The listing builds one solid part. Answer for the finished solid, in the listing's coordinates (mm). A direction names the side the tool comes from. Round coordinates to 2 decimals unless told otherwise and drop trailing zeros. Loops run counter-clockwise (first coordinate to the right, second up) from the corner with the lowest first, then second, coordinate; pieces in that order, holes last. Notation, with made-up numbers: (-32.5, 75) -> (-2.5, 75) arc R20 cw to (-2.5, 107) -> close; hole circle Ø1 at (3.5, 62). An arc over 180 degrees is marked (long way). Use a Markdown table: item, result. Add a question column.
Q1. Given pin 1 Ø7 at (x, z) = (1.5, -4.5) entering from -Y; pin 2 Ø6.5 at (x, z) = (1.5, 168.5) entering from +Y; pin 3 Ø5 at (x, z) = (0.5, 169) entering from -Y, each flat-ended and moving along its own axis, determine where each tip first touches the part or whether it passes through.
Q2. Section B-B on z = 98.5 is taken. Give the vertices of the cut face in (x, y).
Q3. Section A-A on z = -5 is taken. Give the vertices of the cut face in (x, y), then the cut area to 3 significant figures.
Q4. Consider line 1 (Z direction, x = -3.5, y = -7); line 2 (X direction, y = 1.35, z = 167.5); line 3 (Y direction, x = 0.25, z = 140.5). Determine where each line is inside the solid, lowest interval first.
Q5. Which of the six approach directions +Z, -Z, +X, -X, +Y, -Y give full straight-line access (tool end or side, diameter ignored) to faces 5 (the flat face through (0, 4.973, -2)), 6 (the flat face through (0, -4.852, 112)), 7 (the flat face through (7.768, 1, 158))?
Q6. For a pull along Z with two mould halves and no side action, classify faces 1 (the flat face through (0, 1, -9)), 2 (the flat face through (-3, 5, 161)), 3 (the flat face through (0, 8, 70)), 4 (the flat face through (0, 8.648, 158)) as released by +Z, released by -Z, zero draft, split by the parting line, or undercut.
from build123d import *

# Parameters (mm, degrees)
SKETCH2_W           = 23
SKETCH2_H           = 19
BOSS_EXTRUDE1_DEPTH = 70
SKETCH3_W           = 10
SKETCH3_H           = 8
BOSS_EXTRUDE2_DEPTH = 9
SKETCH4_R           = 2
CUT_EXTRUDE1_DEPTH  = 73.156975517
SKETCH5_W           = 12
SKETCH5_H           = 12
BOSS_EXTRUDE3_DEPTH = 85
SKETCH6_W           = 15
SKETCH6_H           = 15
BOSS_EXTRUDE4_DEPTH = 6
BOSS_EXTRUDE5_DEPTH = 10
CUT_EXTRUDE2_START  = -6
CUT_EXTRUDE2_DEPTH  = 6
SKETCH9_R           = 2
CUT_EXTRUDE3_DEPTH  = 172.816281943


with BuildPart() as part:
    # Sketch2 → Boss-Extrude1 (new body)
    with BuildSketch(Plane.XY):
        with Locations((-0.231543624, 1.473154362)):
            Rectangle(SKETCH2_W, SKETCH2_H)
    extrude(amount=BOSS_EXTRUDE1_DEPTH)

    # Sketch3 → Boss-Extrude2 (add)
    with BuildSketch(Plane(origin=(0, 0, 0), x_dir=(-1, 0, 0), z_dir=(0, 0, -1))):
        with Locations((-0.268456376, 0.973154362)):
            Rectangle(SKETCH3_W, SKETCH3_H)
    extrude(amount=BOSS_EXTRUDE2_DEPTH)

    # Sketch4 → Cut-Extrude1 (cut, through all)
    with BuildSketch(Plane(origin=(0, 4.973154362, 0), x_dir=(1, 0, 0), z_dir=(0, 1, 0))):
        with Locations(Location((0.268456376, 5, 0), (0, 0, 180))):
            Circle(SKETCH4_R)
    extrude(amount=-CUT_EXTRUDE1_DEPTH, mode=Mode.SUBTRACT)

    # Sketch5 → Boss-Extrude3 (add)
    with BuildSketch(Plane.XY.offset(70)):
        with Locations((0.268456376, 1.148154362)):
            Rectangle(SKETCH5_W, SKETCH5_H)
    extrude(amount=BOSS_EXTRUDE3_DEPTH)

    # Sketch6 → Boss-Extrude4 (add)
    with BuildSketch(Plane.XY.offset(155)):
        with Locations((0.268456376, 1.148154362)):
            Rectangle(SKETCH6_W, SKETCH6_H)
    extrude(amount=BOSS_EXTRUDE4_DEPTH)

    # Sketch7 → Boss-Extrude5 (add)
    with BuildSketch(Plane.XY.offset(161)):
        with BuildLine():
            ThreePointArc((-4.231543624, 1.148154362), (-2.91352414, -2.033826153), (0.268456376, -3.351845638))
            Line((0.268456376, -3.351845638), (0.268456376, 1.148154362))
            Line((0.268456376, 1.148154362), (-4.231543624, 1.148154362))
        make_face()
        with BuildLine():
            Line((0.268456376, 1.148154362), (0.268456376, -3.351845638))
            ThreePointArc((0.268456376, -3.351845638), (3.450436891, -2.033826153), (4.768456376, 1.148154362))
            Line((4.768456376, 1.148154362), (0.268456376, 1.148154362))
        make_face()
        with BuildLine():
            Line((-4.231543624, 1.148154362), (0.268456376, 1.148154362))
            Line((0.268456376, 1.148154362), (0.268456376, 5.648154362))
            ThreePointArc((0.268456376, 5.648154362), (-2.91352414, 4.330134878), (-4.231543624, 1.148154362))
        make_face()
        with BuildLine():
            Line((0.268456376, 5.648154362), (0.268456376, 1.148154362))
            Line((0.268456376, 1.148154362), (4.768456376, 1.148154362))
            ThreePointArc((4.768456376, 1.148154362), (3.450436891, 4.330134878), (0.268456376, 5.648154362))
        make_face()
        with BuildLine():
            ThreePointArc((-4.231543624, 1.148154362), (-2.91352414, -2.033826153), (0.268456376, -3.351845638))
            Line((0.268456376, -3.351845638), (0.268456376, 1.148154362))
            Line((0.268456376, 1.148154362), (-4.231543624, 1.148154362))
        make_face()
        with BuildLine():
            Line((0.268456376, 1.148154362), (0.268456376, -3.351845638))
            ThreePointArc((0.268456376, -3.351845638), (3.450436891, -2.033826153), (4.768456376, 1.148154362))
            Line((4.768456376, 1.148154362), (0.268456376, 1.148154362))
        make_face()
        with BuildLine():
            Line((-4.231543624, 1.148154362), (0.268456376, 1.148154362))
            Line((0.268456376, 1.148154362), (0.268456376, 5.648154362))
            ThreePointArc((0.268456376, 5.648154362), (-2.91352414, 4.330134878), (-4.231543624, 1.148154362))
        make_face()
        with BuildLine():
            Line((0.268456376, 5.648154362), (0.268456376, 1.148154362))
            Line((0.268456376, 1.148154362), (4.768456376, 1.148154362))
            ThreePointArc((4.768456376, 1.148154362), (3.450436891, 4.330134878), (0.268456376, 5.648154362))
        make_face()
        with BuildLine():
            ThreePointArc((-4.231543624, 1.148154362), (-2.91352414, -2.033826153), (0.268456376, -3.351845638))
            Line((0.268456376, -3.351845638), (0.268456376, 1.148154362))
            Line((0.268456376, 1.148154362), (-4.231543624, 1.148154362))
        make_face()
        with BuildLine():
            Line((0.268456376, 1.148154362), (0.268456376, -3.351845638))
            ThreePointArc((0.268456376, -3.351845638), (3.450436891, -2.033826153), (4.768456376, 1.148154362))
            Line((4.768456376, 1.148154362), (0.268456376, 1.148154362))
        make_face()
        with BuildLine():
            Line((-4.231543624, 1.148154362), (0.268456376, 1.148154362))
            Line((0.268456376, 1.148154362), (0.268456376, 5.648154362))
            ThreePointArc((0.268456376, 5.648154362), (-2.91352414, 4.330134878), (-4.231543624, 1.148154362))
        make_face()
        with BuildLine():
            Line((0.268456376, 5.648154362), (0.268456376, 1.148154362))
            Line((0.268456376, 1.148154362), (4.768456376, 1.148154362))
            ThreePointArc((4.768456376, 1.148154362), (3.450436891, 4.330134878), (0.268456376, 5.648154362))
        make_face()
        with BuildLine():
            ThreePointArc((-4.231543624, 1.148154362), (-2.91352414, -2.033826153), (0.268456376, -3.351845638))
            Line((0.268456376, -3.351845638), (0.268456376, 1.148154362))
            Line((0.268456376, 1.148154362), (-4.231543624, 1.148154362))
        make_face()
        with BuildLine():
            Line((0.268456376, 1.148154362), (0.268456376, -3.351845638))
            ThreePointArc((0.268456376, -3.351845638), (3.450436891, -2.033826153), (4.768456376, 1.148154362))
            Line((4.768456376, 1.148154362), (0.268456376, 1.148154362))
        make_face()
        with BuildLine():
            Line((-4.231543624, 1.148154362), (0.268456376, 1.148154362))
            Line((0.268456376, 1.148154362), (0.268456376, 5.648154362))
            ThreePointArc((0.268456376, 5.648154362), (-2.91352414, 4.330134878), (-4.231543624, 1.148154362))
        make_face()
        with BuildLine():
            Line((0.268456376, 5.648154362), (0.268456376, 1.148154362))
            Line((0.268456376, 1.148154362), (4.768456376, 1.148154362))
            ThreePointArc((4.768456376, 1.148154362), (3.450436891, 4.330134878), (0.268456376, 5.648154362))
        make_face()
    extrude(amount=BOSS_EXTRUDE5_DEPTH)

    # Sketch8 → Cut-Extrude2 (cut)
    with BuildSketch(Plane.XY.offset(171).offset(CUT_EXTRUDE2_START)):
        with BuildLine():
            Line((-3.293495336, 3.898154362), (0.268456376, 3.898154362))
            Line((0.268456376, 3.898154362), (0.268456376, 5.648154362))
            ThreePointArc((0.268456376, 5.648154362), (-1.715857107, 5.187027968), (-3.293495336, 3.898154362))
        make_face()
        with BuildLine():
            Line((0.268456376, 5.648154362), (0.268456376, 3.898154362))
            Line((0.268456376, 3.898154362), (3.830408088, 3.898154362))
            ThreePointArc((3.830408088, 3.898154362), (2.252769859, 5.187027968), (0.268456376, 5.648154362))
        make_face()
        with BuildLine():
            Line((-3.293495336, 3.898154362), (0.268456376, 3.898154362))
            Line((0.268456376, 3.898154362), (0.268456376, 5.648154362))
            ThreePointArc((0.268456376, 5.648154362), (-1.715857107, 5.187027968), (-3.293495336, 3.898154362))
        make_face()
        with BuildLine():
            Line((0.268456376, 5.648154362), (0.268456376, 3.898154362))
            Line((0.268456376, 3.898154362), (3.830408088, 3.898154362))
            ThreePointArc((3.830408088, 3.898154362), (2.252769859, 5.187027968), (0.268456376, 5.648154362))
        make_face()
        with BuildLine():
            ThreePointArc((-3.293495336, -1.601845638), (-1.715857107, -2.890719243), (0.268456376, -3.351845638))
            Line((0.268456376, -3.351845638), (0.268456376, -1.601845638))
            Line((0.268456376, -1.601845638), (-3.293495336, -1.601845638))
        make_face()
        with BuildLine():
            Line((0.268456376, -1.601845638), (0.268456376, -3.351845638))
            ThreePointArc((0.268456376, -3.351845638), (2.252769859, -2.890719243), (3.830408088, -1.601845638))
            Line((3.830408088, -1.601845638), (0.268456376, -1.601845638))
        make_face()
        with BuildLine():
            ThreePointArc((-3.293495336, -1.601845638), (-1.715857107, -2.890719243), (0.268456376, -3.351845638))
            Line((0.268456376, -3.351845638), (0.268456376, -1.601845638))
            Line((0.268456376, -1.601845638), (-3.293495336, -1.601845638))
        make_face()
        with BuildLine():
            Line((0.268456376, -1.601845638), (0.268456376, -3.351845638))
            ThreePointArc((0.268456376, -3.351845638), (2.252769859, -2.890719243), (3.830408088, -1.601845638))
            Line((3.830408088, -1.601845638), (0.268456376, -1.601845638))
        make_face()
    extrude(amount=CUT_EXTRUDE2_DEPTH, mode=Mode.SUBTRACT)

    # Sketch9 → Cut-Extrude3 (cut, through all)
    with BuildSketch(Plane(origin=(0, 3.898154362, 0), x_dir=(1, 0, 0), z_dir=(0, 1, 0))):
        with Locations(Location((0.266504664, -167.5, 0), (0, 0, 180))):
            Circle(SKETCH9_R)
    extrude(amount=-CUT_EXTRUDE3_DEPTH, mode=Mode.SUBTRACT)


solid = part.part
Checked values:
| question | item | result |
|---|---|---|
| 1 | pin 1 | stops at y = -3.03 |
| 1 | pin 2 | stops at y = 3.9 |
| 1 | pin 3 | stops at y = -1.6 |
| 2 | outline | (-5.73, -4.85) -> (6.27, -4.85) -> (6.27, 7.15) -> (-5.73, 7.15) -> close |
| 3 | outline | (-4.73, -3.03) -> (-1.73, -3.03) -> (-1.73, 4.97) -> (-4.73, 4.97) -> close; (2.27, -3.03) -> (5.27, -3.03) -> (5.27, 4.97) -> (2.27, 4.97) -> close |
| 3 | area | 48.0 mm2 |
| 4 | line 1 | z = 0 to 70 |
| 4 | line 2 | x = -4.23 to -1.73, 2.27 to 4.76 |
| 4 | line 3 | y = -4.85 to 7.15 |
| 5 | face 5 | -Z, +X, -X, +Y |
| 5 | face 6 | +X, -X, -Y |
| 5 | face 7 | +Z, +X, +Y, -Y |
| 6 | face 1 | released by -Z |
| 6 | face 2 | released by +Z |
| 6 | face 3 | undercut |
| 6 | face 4 | zero draft |
